from build123d import *

# Parameters (mm, degrees)
EXTRUDE_1_DEPTH      = 20
EXTRUDE_1_DEPTH_BACK = 20
EXTRUDE_2_DEPTH      = 12
EXTRUDE_2_DEPTH_BACK = 12
SKETCH_1_3_W         = 13
SKETCH_1_3_H         = 20
SKETCH_2_W           = 14
SKETCH_2_H           = 6
CUT_EXTRUDE_1_DEPTH  = 8
SKETCH_3_W           = 8
SKETCH_3_H           = 13
CUT_EXTRUDE_2_DEPTH  = 4


with BuildPart() as part:
    # Эскиз1 → Бобышка-Вытянуть1 (new, two sides: drawn at the far end of the back side and taken through both)
    with BuildSketch(Plane.XY.offset(-EXTRUDE_1_DEPTH_BACK)):
        Polygon((-17.5, 5), (-17.5, -25), (17.5, -25), (17.5, 0), (4.5, 0), (4.5, 25), (-17.5, 25), align=None)
    extrude(amount=EXTRUDE_1_DEPTH + EXTRUDE_1_DEPTH_BACK)

    # Эскиз1<3> → Бобышка-Вытянуть2 (add, two sides: drawn at the far end of the back side and taken through both)
    with BuildSketch(Plane.XY.offset(-EXTRUDE_2_DEPTH_BACK)):
        with Locations((-24, 15)):
            Rectangle(SKETCH_1_3_W, SKETCH_1_3_H)
    extrude(amount=EXTRUDE_2_DEPTH + EXTRUDE_2_DEPTH_BACK)

    # Эскиз2 → Вырез-Вытянуть1 (cut)
    with BuildSketch(Plane.XY.offset(20)):
        with Locations((1.5, -22)):
            Rectangle(SKETCH_2_W, SKETCH_2_H)
    extrude(amount=-CUT_EXTRUDE_1_DEPTH, mode=Mode.SUBTRACT)

    # Эскиз3 → Вырез-Вытянуть2 (cut)
    with BuildSketch(Plane(origin=(0, 25, 0), x_dir=(1, 0, 0), z_dir=(0, 1, 0))):
        with Locations((-6.5, 13.5)):
            Rectangle(SKETCH_3_W, SKETCH_3_H)
    extrude(amount=-CUT_EXTRUDE_2_DEPTH, mode=Mode.SUBTRACT)


solid = part.part
Model file for the job. Use its own axes, mm. A direction names the side the tool comes from. Give positions to 0.01 mm unless a question says otherwise; leave off trailing zeros. Order: outer loops, then holes, each group sorted by start corner. A loop starts at its lowest first (then second) coordinate and runs counter-clockwise, first axis right, second up. Notation, with made-up numbers: (71, 80.5) - (105, 80.5) arc R28 ccw to (105, 113.5) - close; hole circle Ø11 at (43.25, 25). An arc over 180 degrees is marked (long way). One line per item, written item: value.
Item 1: Tool access for faces 1 (the flat face through (-24, 15, -12)), 2 (the flat face through (-5.5, -22, 16)), 3 (the flat face through (-24, 5, 0)): list every direction of +Z, -Z, +X, -X, +Y, -Y with a clear straight run to the whole face (end or side of a thin tool).
Response values:
face 1: -Z, -X, +Y, -Y
face 2: +Z, -Y
face 3: +Z, -Z, -X, -Y
Item 2: Slice it at B-B (y = 15). List the corners of the cut face in (x, z).
Response values:
outline: (-30.5, -12) - (-17.5, -12) - (-17.5, -20) - (4.5, -20) - (4.5, 20) - (-17.5, 20) - (-17.5, 12) - (-30.5, 12) - close
Item 3: Pin check, flat tips, straight feed: pin 1 Ø2 at (y, z) = (22, -10.5) entering from +X; pin 2 Ø4 at (x, z) = (10, 8.5) entering from +Y; pin 3 Ø1.2 at (x, y) = (-7, 23) entering from -Z. Stop position of each tip, or through.
Response values:
pin 1: x = 4.5
pin 2: y = 0
pin 3: z = -7
Item 4: Slice it at D-D (z = -8). List the corners of the cut face in (x, y).
Response values:
outline: (-30.5, 5) - (-17.5, 5) - (-17.5, -25) - (17.5, -25) - (17.5, 0) - (4.5, 0) - (4.5, 25) - (-2.5, 25) - (-2.5, 21) - (-10.5, 21) - (-10.5, 25) - (-30.5, 25) - close
Item 5: Slice it at A-A (z = 5.5). List the corners of the cut face in (x, y).
Response values:
outline: (-30.5, 5) - (-17.5, 5) - (-17.5, -25) - (17.5, -25) - (17.5, 0) - (4.5, 0) - (4.5, 25) - (-30.5, 25) - close
Item 6: Slice it at C-C (x = 13.5). List the corners of the cut face in (y, z), then the cut area to 3 significant figures.
Response values:
outline: (-25, -20) - (0, -20) - (0, 20) - (-25, 20) - close
area: 1,000 mm2
Item 7: Two-plate mould, pull along X, no slides. Class faces 4 (the flat face through (17.5, -13, 0)), 5 (the flat face through (1, -19, 16)), 6 (the flat face through (-24, 15, 12)), 7 (the flat face through (8.5, -22, 16)): released by +X, released by -X, zero draft, split by the parting line, or undercut.
Response values:
face 4: released by +X
face 5: undercut
face 6: zero draft
face 7: undercut
Item 8: Wall check: line 1 (X direction, y = 22.5, z = -14); line 2 (X direction, y = 20, z = 4.5); line 3 (X direction, y = -15, z = -17). Give the ranges that are in metal, low to high.
Response values:
line 1: -17.5 to -10.5, -2.5 to 4.5
line 2: -30.5 to 4.5
line 3: -17.5 to 17.5
